The figure shows three views and two pictorial views of one solid part (mm, origin at its lowest corner). Answer the questions. Coordinates: 2 decimals unless noted, no trailing zeros. Loops run counter-clockwise (first coordinate to the right, second up) from the corner with the lowest first, then second, coordinate; pieces in that order, holes last. Notation, with made-up numbers: (-36, 40) -> (-10, 40) arc R29 ccw to (-10, 67) -> close; hole circle Ø4 at (22.5, 44.25). An arc over 180 degrees is marked (long way). Answer as a JSON object with one key per item and string values. Group by question number.
1) Consider probe 1 along X at (y, z) = (14.75, 242.5); probe 2 along Z at (x, y) = (169.5, 5.5) (1 decimal); probe 3 along Z at (x, y) = (176, 1.25) (1 decimal). Determine where each line is inside the solid, lowest interval first. Write a range as [from, to].
2) Section B-B, the plane y = 6.5 is taken. Give the vertices of the cut face in (x, z), plus the area to 3 significant figures.
3) Section A-A, the plane x = 114 is taken. Give the vertices of the cut face in (y, z).
4) Section C-C, the plane z = 200 is taken. Give the vertices of the cut face in (x, y), plus the area to 3 significant figures.
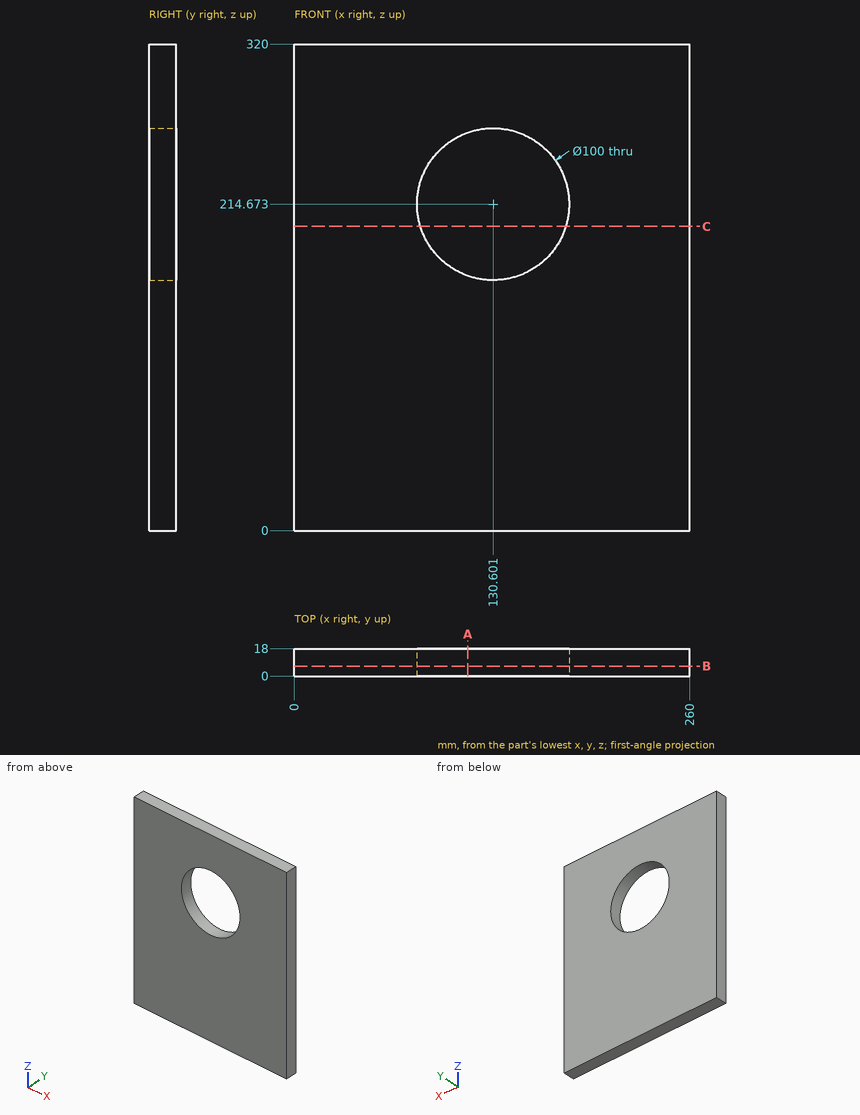
Determined:
{
 "1": {"probe 1": "[0, 89.06], [172.14, 260]", "probe 2": "[0, 183.3], [246.1, 320]", "probe 3": "[0, 193.7], [235.6, 320]"},
 "2": {"outline": "(0, 0) -> (260, 0) -> (260, 320) -> (0, 320) -> close; hole circle Ø100 at (130.6, 214.67)", "area": "75,300 mm²"},
 "3": {"outline": "(0, 0) -> (18, 0) -> (18, 167.51) -> (0, 167.51) -> close; (0, 261.84) -> (18, 261.84) -> (18, 320) -> (0, 320) -> close"},
 "4": {"outline": "(0, 0) -> (82.8, 0) -> (82.8, 18) -> (0, 18) -> close; (178.4, 0) -> (260, 0) -> (260, 18) -> (178.4, 18) -> close", "area": "2,960 mm²"}
}
